The figure shows three views and two pictorial views of one solid part (mm, origin at its lowest corner). Answer the questions. A direction names the side the tool comes from. Round coordinates to 2 decimals unless told otherwise and drop trailing zeros. Order: outer loops, then holes, each group sorted by start corner. A loop starts at its lowest first (then second) coordinate and runs counter-clockwise, first axis right, second up. Notation, with made-up numbers: (77.5, -8) - (132.5, -8) arc R9 cw to (132.5, 3) - close; hole circle Ø5 at (48, 25.5). An arc over 180 degrees is marked (long way). Write item = value, one per line.
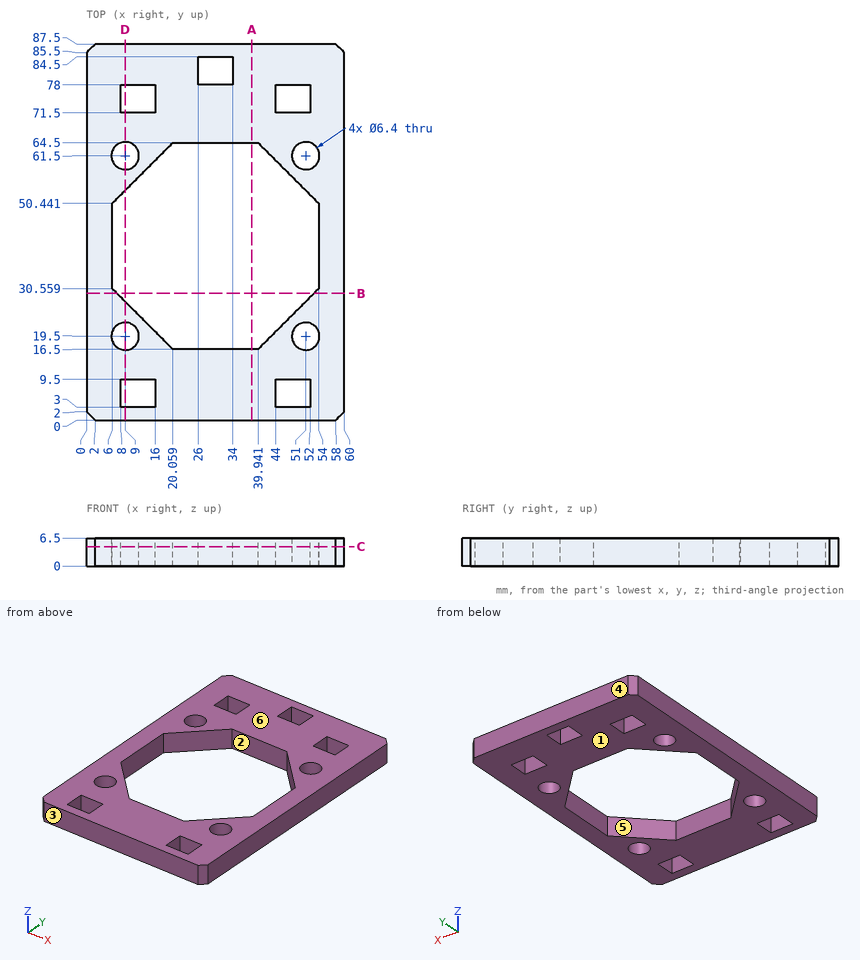
Q1. Section B-B on y = 29.5 is taken. Determine the outline of the cut face in (x, z).
Model answer:
outline = (0, 0) - (7.06, 0) - (7.06, 6.5) - (0, 6.5) - close; (52.94, 0) - (60, 0) - (60, 6.5) - (52.94, 6.5) - close
Q2. Determine the mould class of the marked faces 3, 4, 5 and 6 for opening direction Y: released by +Y, released by -Y, zero draft, split by the parting line, or undercut.
Model answer:
face_3 = released by -Y
face_4 = released by +Y
face_5 = undercut
face_6 = zero draft
Q3. Section D-D on x = 9 is taken. Determine the outline of the cut face in (y, z).
Model answer:
outline = (0, 0) - (3, 0) - (3, 6.5) - (0, 6.5) - close; (9.5, 0) - (16.3, 0) - (16.3, 6.5) - (9.5, 6.5) - close; (22.7, 0) - (27.56, 0) - (27.56, 6.5) - (22.7, 6.5) - close; (53.44, 0) - (58.3, 0) - (58.3, 6.5) - (53.44, 6.5) - close; (64.7, 0) - (71.5, 0) - (71.5, 6.5) - (64.7, 6.5) - close; (78, 0) - (87.5, 0) - (87.5, 6.5) - (78, 6.5) - close
Q4. Flat-ended cylindrical pins translate along their axes: P1, Ø4, axis at x = 45.5, y = 18.5, coming from the -Z side; P2, Ø2, axis at x = 27.5, y = 63, coming from the -Z side. Find the tip coordinate at first contact, or state that the pin passes through.
Model answer:
P1 = 0
P2 = through
Q5. Section C-C on z = 4.5 is taken. Count the separate pieces of the cut face and the enclosed holes in it, then the cut area to 3 significant figures.
Model answer:
separate_pieces = 1
enclosed_holes = 10
area = 2,940 mm^2
Q6. For the marked faces 1 and 2, determine the directions among +Z, -Z, +X, -X, +Y, -Y from which every point of the face is accessible in a straight line to the end or side of a thin tool.
Model answer:
face_1 = -Z, +X, -X, +Y, -Y
face_2 = +Z, -Z
Q7. Section A-A on x = 38.5 is taken. Determine the outline of the cut face in (y, z), then the cut area to 3 significant figures.
Model answer:
outline = (0, 0) - (16.5, 0) - (16.5, 6.5) - (0, 6.5) - close; (64.5, 0) - (87.5, 0) - (87.5, 6.5) - (64.5, 6.5) - close
area = 257 mm^2
Q8. Find the intervals of material crossed by line 1 (X direction, y = 5.5, z = 0.5); line 2 (X direction, y = 47, z = 5.75); line 3 (Y direction, x = 37, z = 1.25), in increasing order. Write a range as from..to.
Model answer:
line_1 = 0..8, 16..44, 52..60
line_2 = 0..6, 54..60
line_3 = 0..16.5, 64.5..87.5
